The listing builds one solid part. Answer for the finished solid, in the listing's coordinates (mm). Round coordinates to 2 decimals unless told otherwise and drop trailing zeros. Write each loop counter-clockwise with the first axis right and the second up, starting at its lowest first coordinate (ties: lowest second). Pieces come first, ordered by that corner, then holes.
(1) A cutting plane is placed at A-A, the plane z = 1.55. Give the number of separate pieces and of enclosed holes in the cut face, and give its area (3 significant figures).
(2) A cutting plane is placed at B-B, the plane x = 54. Give the vertices of the cut face in (y, z) (3 decimals).
(3) The mould has two halves that part along Y. Classify faces 1 (the face through (65.969, 176.146, 1.565)), 2 (the face through (-3.097, 201.952, 1.565)), 3 (the face through (-34.917, 216.668, 1.565)): +Y half, -Y half, draft (parallel to the pull), parting line (faces both ways), or undercut.
(4) Each of these flat-tipped pins is pushed along its axis until it touches: pin 1 Ø1 at (x, z) = (116.5, 2.5) entering from -Y (3 decimals); pin 2 Ø1.5 at (x, z) = (277.5, 2.5) entering from -Y; pin 3 Ø1.5 at (y, z) = (230.5, 1.5) entering from +X; pin 4 Ø17 at (x, y) = (0, 215.9) entering from +Z (1 decimal). Where does it stop, or does it pass through?
(5) Find the intervals of material crossed by probe 1 along Y at (x, z) = (19, 1.25) (3 decimals); probe 2 along Y at (x, z) = (0, 1.5) (1 decimal); probe 3 along X at (y, z) = (75, 2.95), in increasing order.
(6) A cutting plane is placed at C-C, the plane y = 112. Give the vertices of the cut face in (x, z) (3 decimals).
from build123d import *

# Parameters (mm, degrees)
SKETCH1_R           = 14.2875
BOSS_EXTRUDE1_DEPTH = 3.175


with BuildPart() as part:
    # Sketch1 → Boss-Extrude1 (new body)
    with BuildSketch(Plane.XY):
        with BuildLine():
            Line((134.62, 180.975), (142.401211704, 69.698488351))
            ThreePointArc((142.401211704, 69.698488351), (155.003963594, 51.188868036), (177.319809019, 53.043171796))
            Line((177.319809019, 53.043171796), (307.36019605, 144.098431067))
            ThreePointArc((307.36019605, 144.098431067), (316.647321796, 159.403140629), (311.6377975, 176.590039876))
            Line((311.6377975, 176.590039876), (279.800527192, 214.532221144))
            ThreePointArc((279.800527192, 214.532221144), (244.908427164, 241.305871163), (201.970411771, 250.825))
            Line((201.970411771, 250.825), (0, 250.825))
            ThreePointArc((0, 250.825), (-34.925, 215.9), (0, 180.975))
            Line((0, 180.975), (25.4, 180.975))
            Line((25.4, 180.975), (35.56, 171.45))
            Line((35.56, 171.45), (60.96, 171.45))
            Line((60.96, 171.45), (71.12, 180.975))
            Line((71.12, 180.975), (134.62, 180.975))
        make_face()
        with Locations((294.612459752, 162.304085251)):
            Circle(SKETCH1_R, mode=Mode.SUBTRACT)
        with Locations((164.572072721, 71.24882598)):
            Circle(SKETCH1_R, mode=Mode.SUBTRACT)
        with Locations((0, 215.9)):
            Circle(SKETCH1_R, mode=Mode.SUBTRACT)
    extrude(amount=BOSS_EXTRUDE1_DEPTH)


solid = part.part
Solutions:
1. separate pieces: 1
1. enclosed holes: 3
1. area: 35,400 mm2
2. outline: (171.45, 0) - (250.825, 0) - (250.825, 3.175) - (171.45, 3.175) - close
3. face 1: -Y half
3. face 2: undercut
3. face 3: parting line
4. pin 1: stops at y = 180.975
4. pin 2: stops at y = 122.66
4. pin 3: stops at x = 263.92
4. pin 4: passes through
5. probe 1: y = 180.975 to 250.825
5. probe 2: y = 181 to 201.6, 230.2 to 250.8
5. probe 3: x = 142.03 to 150.79, 178.36 to 208.68
6. outline: (139.443, 0) - (261.519, 0) - (261.519, 3.175) - (139.443, 3.175) - close
